Work out the finished part from the listing and answer in its coordinate system (mm). Round coordinates to 2 decimals unless told otherwise and drop trailing zeros. Order: outer loops, then holes, each group sorted by start corner. A loop starts at its lowest first (then second) coordinate and runs counter-clockwise, first axis right, second up. Notation, with made-up numbers: (66, 15.5) - (103, 15.5) arc R14 ccw to (103, 39.5) - close; hole circle Ø10 at (-34, 54). An arc over 180 degrees is marked (long way). Use one line per item in the form item = value. Start each with the question number.
Q1. Find the intervals of material crossed by line 1 (Y direction, x = -107, z = 1.75); line 2 (X direction, y = 43, z = 3.55); line 3 (Y direction, x = 37.5, z = 4), in increasing order. Write a range as [from, to].
Q2. The part is cut by section A-A on z = 4.2. Determine the outline of the cut face in (x, y), plus the area to 3 significant figures.
Q3. The part is cut by section B-B on x = -46.5. Determine the outline of the cut face in (y, z), plus the area to 3 significant figures.
Q4. Given P1, Ø2.5, axis at y = -52, z = 3.5, coming from the +X side; P2, Ø3, axis at x = 36, z = 4.5, coming from the +Y side; P3, Ø1.5, axis at y = -51.5, z = 2.5, coming from the -X side, each flat-ended and moving along its own axis, determine where each tip first touches the part or whether it passes through.
Q5. The part is cut by section C-C on y = 42.5. Determine the outline of the cut face in (x, z).
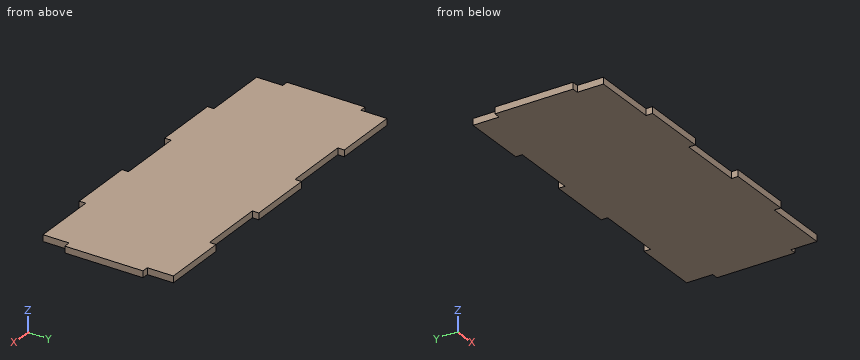
Autodesk Inventor part; units mm, degrees
ref_plane "YZ Plane" through (0, 0, 0) normal (1, 0, 0) x (0, 1, 0)
ref_plane "XZ Plane" through (0, 0, 0) normal (0, 1, 0) x (-1, 0, 0)
ref_plane "XY Plane" through (0, 0, 0) normal (0, 0, 1) x (1, 0, 0)
sketch "Sketch1" plane through (0, 0, 0) normal (0, 0, 1) x (1, 0, 0)
  line L0 (-130, -50) -> (130, -50)
  line L1 (130, -50) -> (130, 50)
  line L2 (130, 50) -> (-130, 50)
  line L3 (-130, 50) -> (-130, -50)
  line L4 (-130, -50) -> (130, 50) construction
  line L5 (130, -50) -> (-130, 50) construction
  line L6 (-75, -50) -> (-25, -50)
  line L7 (-25, -50) -> (-25, -55)
  line L8 (-25, -55) -> (-75, -55)
  line L9 (-75, -55) -> (-75, -50)
  line L10 (25, -50) -> (75, -50)
  line L11 (75, -50) -> (75, -55)
  line L12 (75, -55) -> (25, -55)
  line L13 (25, -55) -> (25, -50)
  line L14 (130, 50) -> (125, 50)
  line L15 (125, 50) -> (125, 30)
  line L16 (125, 30) -> (130, 30)
  line L17 (130, 30) -> (130, 50)
  line L18 (130, -50) -> (125, -50)
  line L19 (125, -50) -> (125, -30)
  line L20 (125, -30) -> (130, -30)
  line L21 (130, -30) -> (130, -50)
  line L22 (0, 50) -> (0, -50) construction
  line L23 (-125, 50) -> (-125, 30)
  line L24 (-125, 30) -> (-130, 30)
  line L25 (-125, -50) -> (-125, -30)
  line L26 (-125, -30) -> (-130, -30)
  line L27 (-75, 50) -> (-25, 50)
  line L28 (-25, 50) -> (-25, 45)
  line L29 (-25, 45) -> (-75, 45)
  line L30 (-75, 45) -> (-75, 50)
  line L31 (25, 50) -> (75, 50)
  line L32 (75, 50) -> (75, 45)
  line L33 (75, 45) -> (25, 45)
  line L34 (25, 45) -> (25, 50)
  point P0 (0, 0)
  point P1 (-75, -52.5)
  point P2 (-25, -50)
  point P3 (75, -50)
  point P4 (-125, -50)
  point P5 (130, -30)
  point P6 (130, 30)
  point P7 (125, 50)
  point P8 (-125, 50)
  point P9 (-130, 30)
  point P10 (75, 50)
  point P11 (-25, 50)
  dimension "d0" = 260
  dimension "d1" = 100
  dimension "d2" = 50
  dimension "d3" = 50
  dimension "d4" = 50
  dimension "d5" = 55
  dimension "d6" = 5
  dimension "d10" = 20
  dimension "d12" = 5
  dimension "d13" = 50
  dimension "d14" = 50
  dimension "d15" = 5
  dimension "d16" = 20
extrude "Extrusion1" add sketch "Sketch1" along normal blind 5 contours L25 L26 L3 L24 L23 L2 L30 L29 L28 L34 L33 L32 L15 L16 L1 L20 L19 L0 | L0 L7 L8 L9 | L0 L11 L12 L13
equation "\"BendRadius\" = Thickness"
equation "\"BendReliefWidth\" = Thickness"
equation "\"BendReliefDepth\" = 0.5 * Thickness"
equation "\"CornerReliefSize\" = 4 * Thickness"
equation "\"MinimumRemnant\" = 2 * Thickness"
equation "\"TransitionRadius\" = BendRadius"
equation "\"JacobiRadiusSize\" = BendRadius"
equation "\"GapSize\" = Thickness"
properties part number "Lat1(2)" material "Wood (Cherry)"
Found:
q1.line_1 = [-50, 50]
q1.line_2 = [-125, 125]
q1.line_3 = [-55, 45]
q2.outline = (-130, -30) - (-125, -30) - (-125, -50) - (-75, -50) - (-75, -55) - (-25, -55) - (-25, -50) - (25, -50) - (25, -55) - (75, -55) - (75, -50) - (125, -50) - (125, -30) - (130, -30) - (130, 30) - (125, 30) - (125, 50) - (75, 50) - (75, 45) - (25, 45) - (25, 50) - (-25, 50) - (-25, 45) - (-75, 45) - (-75, 50) - (-125, 50) - (-125, 30) - (-130, 30) - close
q2.area = 25,600 mm²
q3.outline = (-55, 0) - (45, 0) - (45, 5) - (-55, 5) - close
q3.area = 500 mm²
q4.P1 = 75
q4.P2 = 45
q4.P3 = -75
q5.outline = (-125, 0) - (125, 0) - (125, 5) - (-125, 5) - close
